Source: CAD feature listing. Evaluate the final solid. Frame: model axes, mm. A direction names the side the tool comes from. Round coordinates to 2 decimals unless told otherwise and drop trailing zeros. Write each loop counter-clockwise with the first axis right and the second up, starting at its lowest first coordinate (ties: lowest second). Pieces come first, ordered by that corner, then holes. Notation, with made-up numbers: M 25.25,77.25 L 62.25,77.25 A8 cw 62.25,84.25 Z; hole C 49.5,-34.5 d11. An arc over 180 degrees is marked long. Answer in a Markdown table with one row per item.
Autodesk Inventor part; units mm, degrees
ref_plane "YZ Plane" through (0, 0, 0) normal (1, 0, 0) x (0, 1, 0)
ref_plane "XZ Plane" through (0, 0, 0) normal (0, 1, 0) x (-1, 0, 0)
ref_plane "XY Plane" through (0, 0, 0) normal (0, 0, 1) x (1, 0, 0)
sketch "Sketch1" plane through (0, 0, 0) normal (0, 0, 1) x (1, 0, 0)
  circle A0 centre (0, 0) radius 2.0828
  dimension "d0" = 4.1656
extrude "Extrusion1" add sketch "Sketch1" along normal blind 31.75
sketch "Sketch2" plane through (0, 0, 0) normal (0, 1, 0) x (-1, 0, 0)
  line L0 (0, 0) -> (0, -2.2098)
  line L1 (0, 0) -> (3.9624, 0)
  line L2 (0, -2.2098) -> (2.032, -2.2098)
  line L3 (3.9624, 0) -> (3.9624, 3.6562) construction
  arc A0 (2.032, -2.2098) -> (3.9624, -0.4599) centre (0.1837, 1.7689) ccw
  line L4 (4.5847, 0.6553) -> (4.5847, -0.2608) construction
  line L5 (3.9624, -0.4599) -> (3.9624, 0)
  dimension "d3" = 2.2098
  dimension "d6" = 2.032
  dimension "d19" = 3.9624
revolve "Revolution1" add sketch "Sketch2" angle 360 about axis through (0, 0, 0) along (0, 0, -1)
sketch "Sketch3" plane through (0, 0, -2.2098) normal (0, 0, -1) x (-1, 0, 0)
  circle A0 centre (0, 0) radius 2.032
  line L0 (-0.6874, 1.1906) -> (0.6874, 1.1906)
  line L1 (0.6874, 1.1906) -> (1.3748, 0)
  line L2 (1.3748, 0) -> (0.6874, -1.1906)
  line L3 (0.6874, -1.1906) -> (-0.6874, -1.1906)
  line L4 (-0.6874, -1.1906) -> (-1.3748, 0)
  line L5 (-1.3748, 0) -> (-0.6874, 1.1906)
  dimension "d8" = 2.3813
extrude "Extrusion2" cut sketch "Sketch3" against normal blind 1.5875 contours L0 L1 L2 L3 L4 L5
chamfer "Chamfer1" distance 0.508 angle 45 1 edges at (-2.0828, 0, 31.75)
thread "Thread1"
properties part number "10-32 x500 button head" material "Steel"
Q1. Section A-A (z = 12.5). Return loops of the section in (x, y), and give its area (3 significant figures).
Solutions:
| item | result |
|---|---|
| outline | C 0,0 d4.17 |
| area | 13.6 mm2 |
Q2. Access query for faces 4 (the flat face through (-1.03, 0.6, -1.43)), 5 (the flat face through (0, 0, 31.75)). Directions: +Z, -Z, +X, -X, +Y, -Y. A direction counts if a zero-diameter tool reaches every point of the face in a straight line with its end or side. Return the directions, or none.
Solutions:
| item | result |
|---|---|
| face 4 | -Z |
| face 5 | +Z, +X, -X, +Y, -Y |
Q3. Pull-direction query (Y, two-part tool) for faces 1 (the flat face through (0, 1.191, -1)), 2 (the flat face through (-2, -2, 0)), 3 (the cylindrical face through (1.987, -0.626, 15.402)); classes: pulls with the +Y half, pulls with the -Y half, needs draft (parallel to the pull), parting line crosses it, or undercut.
Solutions:
| item | result |
|---|---|
| face 1 | undercut |
| face 2 | needs draft |
| face 3 | parting line crosses it |
Q4. Contact query for flat-ended pins moving along their axis: pin 1 Ø0.7 at (x, z) = (0, -1.5) entering from +Y; pin 2 Ø3 at (x, y) = (2, -2.5) entering from +Z; pin 3 Ø1.5 at (x, z) = (-2, 20) entering from +Y. Output: stop coordinate, or through.
Solutions:
| item | result |
|---|---|
| pin 1 | stops at y = 3.46 |
| pin 2 | stops at z = 31.62 |
| pin 3 | stops at y = 1.67 |
Q5. Material intervals for probe 1 along Z at (x, y) = (0.75, 0.5); probe 2 along Z at (x, y) = (2.25, 0.75); probe 3 along X at (y, z) = (0.25, 11), sorted ascending.
Solutions:
| item | result |
|---|---|
| probe 1 | z = -0.62 to 31.75 |
| probe 2 | z = -2.03 to 0 |
| probe 3 | x = -2.07 to 2.07 |
